Design review of the part built by this model. Coordinates are the model's own, in mm. A direction names the side the tool comes from. Round coordinates to 2 decimals unless told otherwise and drop trailing zeros. Write each loop counter-clockwise with the first axis right and the second up, starting at its lowest first coordinate (ties: lowest second). Pieces come first, ordered by that corner, then holes. Notation, with made-up numbers: (77.25, 24) -> (136.25, 24) arc R14 cw to (136.25, 44) -> close; hole circle Ø9 at (75, 28.25). An arc over 180 degrees is marked (long way). Write item = value, one per line. Start each with the question number.
Item 1: Add section D-D, the plane z = -22.5. State the section outline as (x, y) points.
Item 2: Mouldability with a two-part tool opening along Z and no side actions: class faces 3 (the flat face through (-1, 0, 15)), 4 (the flat face through (3, 1.5, -1)), 5 (the cylindrical face through (-55.55, 2.465, 42.594)) as released by +Z, released by -Z, zero draft, split by the parting line, or undercut.
Item 3: Machinability: for faces 1 (the cylindrical face through (-37.11, 3.26, 47.42)), 2 (the cylindrical face through (-29.715, 0.76, 50.093)), which of the approach directions +Z, -Z, +X, -X, +Y, -Y give a long, thin tool a straight path to every point of the face, cutting with its end or side? Answer none if there is none.
Item 4: For pin 1 Ø6 at (x, z) = (-50, -30.5) entering from +Y; pin 2 Ø2 at (x, y) = (29, 2.5) entering from -Z; pin 3 Ø5 at (x, z) = (33.04, -50.64) entering from +Y; pin 4 Ø3 at (y, z) = (3.5, -48.5) entering from +X, all flat-tipped, find the tip position at first contact; note any pin that passes through.
Item 5: To check wall thickness, follow L1, parallel to Z at x = 52, y = 1.7; L2, parallel to Z at x = -2.5, y = 2.85 (3 decimals); L3, parallel to X at y = 2.3, z = -31. State the ranges of each line that lie inside material, in increasing order.
Item 6: Add section C-C, the plane y = 3.6. State the section outline as (x, z) points.
Item 7: Add section A-A, the plane z = 0. State the section outline as (x, y) points (3 decimals), then the cut area to 3 significant figures.
Item 8: Add section B-B, the plane x = 0. State the section outline as (y, z) points (3 decimals).
from build123d import *

# Parameters (mm, degrees)
SKETCH1_R           = 70
BOSS_EXTRUDE1_DEPTH = 5
CIRPATTERN1_COUNT   = 4


with BuildPart() as part:
    # Sketch1 → Boss-Extrude1 (new body)
    with BuildSketch(Plane(origin=(0, 0, 0), x_dir=(1, 0, 0), z_dir=(0, 1, 0))):
        Circle(SKETCH1_R)
    extrude(amount=BOSS_EXTRUDE1_DEPTH)

    # Sketch3 → CBORE for M5 Hex Head Bolt1 (revolve, cut)
    with BuildSketch(Plane(origin=(-50.502701159, 5, -32.395635133), x_dir=(0, 0, 1), z_dir=(1, 0, 0))):
        Polygon((0, 0), (0, 5), (2.75, 5), (2.75, 3.5), (6.119, 3.5), (6.119, 0.025), (6.144, 0), align=None)
    cbore_for_m5_hex_head_bolt1 = revolve(axis=Axis((-50.502701159, 11.35, -32.395635133), (0, -1, 0)), mode=Mode.SUBTRACT)

    # CirPattern1: CBORE for M5 Hex Head Bolt1 ×4 about axis
    cirpattern1_axis = Axis((0.392084454, 0, 0.251507833), (0, 1, 0))
    for i in range(1, CIRPATTERN1_COUNT):
        add(cbore_for_m5_hex_head_bolt1.rotate(cirpattern1_axis, i * 360 / CIRPATTERN1_COUNT), mode=Mode.SUBTRACT)

    # Sketch7 → CBORE for M5 Hex Head Bolt2 (revolve, cut)
    with BuildSketch(Plane(origin=(0, 5, 0), x_dir=(0, 0, 1), z_dir=(1, 0, 0))):
        Polygon((0, 0), (0, 5), (2.75, 5), (2.75, 3.5), (6.119, 3.5), (6.119, 0.025), (6.144, 0), align=None)
    revolve(axis=Axis((0, 11.35, 0), (0, -1, 0)), mode=Mode.SUBTRACT)


solid = part.part
Result set:
q1.outline = (-66.29, 0) -> (66.29, 0) -> (66.29, 5) -> (-66.29, 5) -> close
q2.face_3 = zero draft
q2.face_4 = undercut
q2.face_5 = split by the parting line
q3.face_1 = +Y
q3.face_2 = +Y, -Y
q4.pin_1 = 1.5
q4.pin_2 = -64.16
q4.pin_3 = through
q4.pin_4 = 51.87
q5.L1 = -46.86 to 26.82, 38.98 to 46.86
q5.L2 = -69.955 to -5.585, 5.585 to 69.955
q5.L3 = -62.76 to -56.46, -44.54 to 62.76
q6.outline = circle Ø140 at (0, 0); hole circle Ø12.24 at (-50.5, -32.4); hole circle Ø12.24 at (-32.26, 51.15); hole circle Ø12.24 at (0, 0); hole circle Ø12.24 at (33.04, -50.64); hole circle Ø12.24 at (51.29, 32.9)
q7.outline = (-70, 0) -> (-2.75, 0) -> (-2.75, 1.5) -> (-6.119, 1.5) -> (-6.119, 4.975) -> (-6.144, 5) -> (-70, 5) -> close; (2.75, 0) -> (70, 0) -> (70, 5) -> (6.144, 5) -> (6.119, 4.975) -> (6.119, 1.5) -> (2.75, 1.5) -> close
q7.area = 649 mm²
q8.outline = (0, -70) -> (5, -70) -> (5, -6.144) -> (4.975, -6.119) -> (1.5, -6.119) -> (1.5, -2.75) -> (0, -2.75) -> close; (0, 2.75) -> (1.5, 2.75) -> (1.5, 6.119) -> (4.975, 6.119) -> (5, 6.144) -> (5, 70) -> (0, 70) -> close
